Drawing for the job (mm, zero at the part's lowest x, y, z). Round coordinates to 2 decimals unless told otherwise and drop trailing zeros. Order: outer loops, then holes, each group sorted by start corner. A loop starts at its lowest first (then second) coordinate and runs counter-clockwise, first axis right, second up. Notation, with made-up numbers: (42.5, 43.25) - (81.5, 43.25) arc R16 ccw to (81.5, 54.25) - close; hole circle Ø6 at (26, -3.5). An arc over 180 degrees is marked (long way). Put each result on its own line as item: value. Start each with the question number.
Item 1: Saw through at D-D on z = 7.5. List the corners of the cut face in (x, y).
Item 2: Saw through at B-B on y = 1.15. List the corners of the cut face in (x, z).
Item 3: Probe probe 1 along X at (y, z) = (0.75, 20.32); probe 2 along Z at (x, y) = (35, 1.3); probe 3 along Z at (x, y) = (3, 1.05). List the from-to ranges inside material, lowest first.
Item 4: Saw through at C-C on z = 1.75. List the corners of the cut face in (x, y).
Item 5: Pin check, flat tips, straight feed: pin 1 Ø8 at (x, z) = (33, 4) entering from -Y; pin 2 Ø0.5 at (y, z) = (0.5, 8.5) entering from -X; pin 3 Ø1 at (y, z) = (1, 11.5) entering from +X. Stop position of each tip, or through.
Item 6: Saw through at A-A on z = 20.32. List the corners of the cut face in (x, y), plus the area to 3 significant figures.
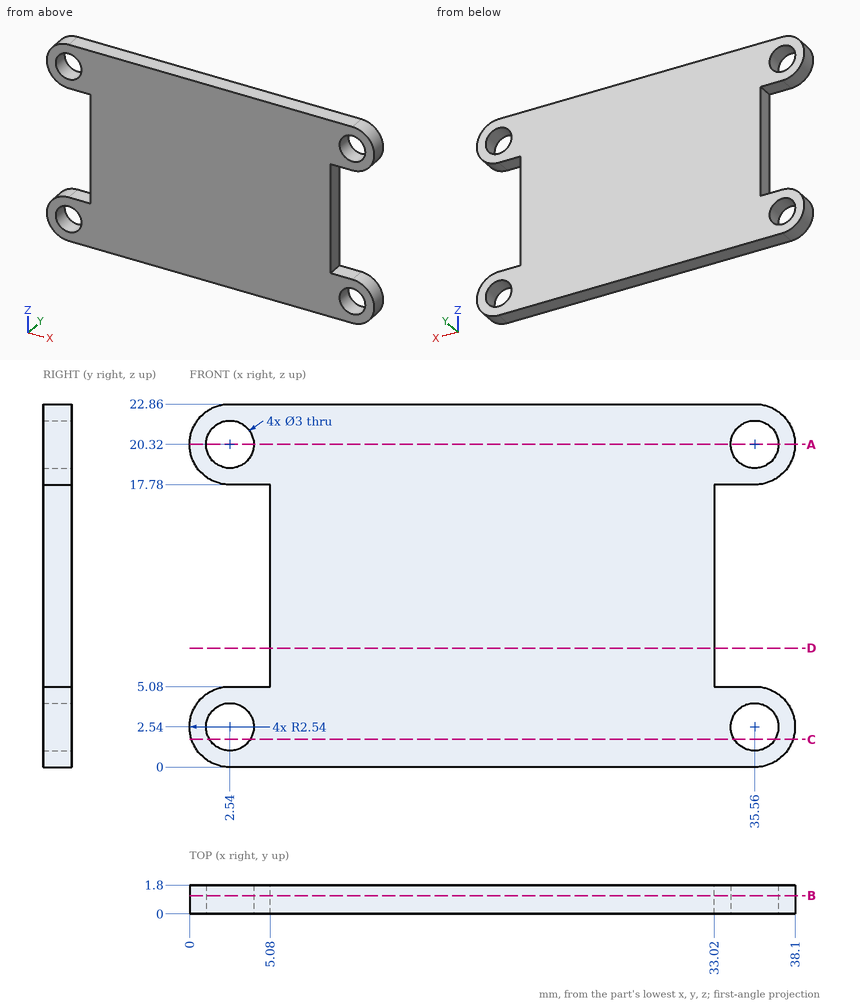
Results found:
1. outline: (5.08, 0) - (33.02, 0) - (33.02, 1.8) - (5.08, 1.8) - close
2. outline: (2.54, 0) - (35.56, 0) arc R2.54 ccw to (35.56, 5.08) - (33.02, 5.08) - (33.02, 17.78) - (35.56, 17.78) arc R2.54 ccw to (35.56, 22.86) - (2.54, 22.86) arc R2.54 ccw to (2.54, 17.78) - (5.08, 17.78) - (5.08, 5.08) - (2.54, 5.08) arc R2.54 ccw to start; hole circle Ø3 at (2.54, 2.54); hole circle Ø3 at (2.54, 20.32); hole circle Ø3 at (35.56, 2.54); hole circle Ø3 at (35.56, 20.32)
3. probe 1: x = 0 to 1.04, 4.04 to 34.06, 37.06 to 38.1
3. probe 2: z = 0 to 1.15, 3.93 to 5.08, 17.78 to 18.93, 21.71 to 22.86
3. probe 3: z = 0 to 1.11, 3.97 to 5.08, 17.78 to 18.89, 21.75 to 22.86
4. outline: (0.13, 0) - (1.26, 0) - (1.26, 1.8) - (0.13, 1.8) - close; (3.82, 0) - (34.28, 0) - (34.28, 1.8) - (3.82, 1.8) - close; (36.84, 0) - (37.97, 0) - (37.97, 1.8) - (36.84, 1.8) - close
5. pin 1: stops at y = 0
5. pin 2: stops at x = 5.08
5. pin 3: stops at x = 33.02
6. outline: (0, 0) - (1.04, 0) - (1.04, 1.8) - (0, 1.8) - close; (4.04, 0) - (34.06, 0) - (34.06, 1.8) - (4.04, 1.8) - close; (37.06, 0) - (38.1, 0) - (38.1, 1.8) - (37.06, 1.8) - close
6. area: 57.8 mm²
